Model file for the job. Use its own axes, mm. Face numbers are marked on the shaded views. A direction names the side the tool comes from. Give positions to 0.01 mm unless a question says otherwise; leave off trailing zeros. Loops run counter-clockwise (first coordinate to the right, second up) from the corner with the lowest first, then second, coordinate; pieces in that order, holes last. Notation, with made-up numbers: (-25.5, -37) -> (-3.5, -37) arc R16 ccw to (-3.5, -18) -> close; hole circle Ø10 at (-1.75, 74). An arc over 180 degrees is marked (long way). Use CSV: the item, a comma, the result in double quotes. Start each with the question number.
(1) Cut at A-A on x = 17. Write the cut outline in (y, z).
(2) Cut at D-D on z = 11. Write the cut outline in (x, y), then the cut area to 3 significant figures.
(3) Pull direction X, two halves, no side cores. Call the marked faces 3, 4 and 5: pulls with the +X half, pulls with the -X half, needs draft (parallel to the pull), parting line crosses it, or undercut.
(4) Flat gauge pins, fed straight in: pin 1 (2.5 mm diameter, centred on x = -15, z = -10, fed in from +Y); pin 2 (5.5 mm diameter, centred on x = -14.5, z = 11, fed in from -Y); pin 3 (5 mm diameter, centred on y = 14.5, z = -11.5, fed in from -X); pin 4 (8.5 mm diameter, centred on x = 7, z = -1, fed in from +Y). Where does each tip first touch, or does it go through?
(5) Cut at C-C on x = -14.5. Write the cut outline in (y, z), then the cut area to 3 significant figures.
(6) Drill centre lines: probe 1 along Z at (x, y) = (-8, 11); probe 2 along X at (y, z) = (1.5, 2.5); probe 3 along X at (y, z) = (1, -11). Where is each one in solid material? Low to high.
(7) 3-axis set-ups, long thin cutter, end or side, ignore diameter. For the marked faces 1 and 2: which of +Z, -Z, +X, -X, +Y, -Y reach the whole face in a straight line?
(8) Cut at B-B on y = 10.5. Write the cut outline in (x, z), then the cut area to 3 significant figures.
from build123d import *

# Parameters (mm, degrees)
SKETCH1_W           = 42
SKETCH1_H           = 28
BOSS_EXTRUDE1_DEPTH = 17
BOSS_EXTRUDE3_DEPTH = 0.8
SKETCH4_R           = 1.65
CUT_EXTRUDE1_DEPTH  = 10.8
SKETCH5_W           = 10
SKETCH5_H           = 5
CUT_EXTRUDE2_DEPTH  = 10.8
FILLET1_R           = 1.5
BOSS_EXTRUDE4_START = 1.5
SKETCH6_R           = 2.65
SKETCH6_R_2         = 1.65
BOSS_EXTRUDE4_DEPTH = 1.5


with BuildPart() as part:
    # Sketch1 → Boss-Extrude1 (new body)
    with BuildSketch(Plane(origin=(0, 0, 0), x_dir=(1, 0, 0), z_dir=(0, 1, 0))):
        Polygon((-22, 15), (-23.5, 4.326945416), (-23.5, -4.326945416), (-22, -15), (22, -15), (23.5, -4.326945416), (23.5, 4.326945416), (22, 15), align=None)
        Rectangle(SKETCH1_W, SKETCH1_H, mode=Mode.SUBTRACT)
    extrude(amount=BOSS_EXTRUDE1_DEPTH)

    # Sketch3 → Boss-Extrude3 (add)
    with BuildSketch(Plane.XZ):
        Polygon((-22, 15), (22, 15), (23.5, 4.326945416), (23.5, -4.326945416), (22, -15), (-22, -15), (-23.5, -4.326945416), (-23.5, 4.326945416), align=None)
    extrude(amount=BOSS_EXTRUDE3_DEPTH)

    # Sketch4 → Cut-Extrude1 (cut)
    with BuildSketch(Plane(origin=(0, 0, 0), x_dir=(1, 0, 0), z_dir=(0, 1, 0))):
        with Locations(Location((-14.5, 11, 0), (0, 0, 270))):
            Circle(SKETCH4_R)
        with Locations(Location((7.8, 11.302833977, 0), (0, 0, 270))):
            Circle(SKETCH4_R)
        with Locations(Location((-14.5, -11, 0), (0, 0, 270))):
            Circle(SKETCH4_R)
        with Locations(Location((7.8, -11.16509614, 0), (0, 0, 270))):
            Circle(SKETCH4_R)
    extrude(amount=-CUT_EXTRUDE1_DEPTH, mode=Mode.SUBTRACT)

    # Sketch5 → Cut-Extrude2 (cut)
    with BuildSketch(Plane.XY.offset(-14)):
        with Locations((16, 4)):
            Rectangle(SKETCH5_W, SKETCH5_H)
    extrude(amount=-CUT_EXTRUDE2_DEPTH, mode=Mode.SUBTRACT)

    # Fillet1
    fillet1_edges = [part.edges().sort_by_distance(p)[0] for p in [
        (11, 1.5, -14.5),
        (11, 6.5, -14.5),
    ]]
    fillet(fillet1_edges, radius=FILLET1_R)

    # Sketch6 → Boss-Extrude4 (add)
    # profile 1 of 4: a face of its own
    with BuildSketch(Plane(origin=(0, 0, 0), x_dir=(1, 0, 0), z_dir=(0, 1, 0)).offset(BOSS_EXTRUDE4_START)):
        with Locations(Location((-14.5, 11, 0), (0, 0, 270))):
            Circle(SKETCH6_R)
        with Locations(Location((-14.5, 11, 0), (0, 0, 270))):
            Circle(SKETCH6_R_2, mode=Mode.SUBTRACT)
    # profile 2 of 4: a face of its own
    with BuildSketch(Plane(origin=(0, 0, 0), x_dir=(1, 0, 0), z_dir=(0, 1, 0)).offset(BOSS_EXTRUDE4_START)):
        with Locations(Location((7.8, 11.302833977, 0), (0, 0, 270))):
            Circle(SKETCH6_R)
        with Locations(Location((7.8, 11.302833977, 0), (0, 0, 270))):
            Circle(SKETCH6_R_2, mode=Mode.SUBTRACT)
    # profile 3 of 4: a face of its own
    with BuildSketch(Plane(origin=(0, 0, 0), x_dir=(1, 0, 0), z_dir=(0, 1, 0)).offset(BOSS_EXTRUDE4_START)):
        with Locations(Location((7.8, -11.16509614, 0), (0, 0, 270))):
            Circle(SKETCH6_R)
        with Locations(Location((7.8, -11.16509614, 0), (0, 0, 270))):
            Circle(SKETCH6_R_2, mode=Mode.SUBTRACT)
    # profile 4 of 4: a face of its own
    with BuildSketch(Plane(origin=(0, 0, 0), x_dir=(1, 0, 0), z_dir=(0, 1, 0)).offset(BOSS_EXTRUDE4_START)):
        with Locations(Location((-14.5, -11, 0), (0, 0, 270))):
            Circle(SKETCH6_R)
        with Locations(Location((-14.5, -11, 0), (0, 0, 270))):
            Circle(SKETCH6_R_2, mode=Mode.SUBTRACT)
    extrude(amount=-BOSS_EXTRUDE4_DEPTH)


solid = part.part
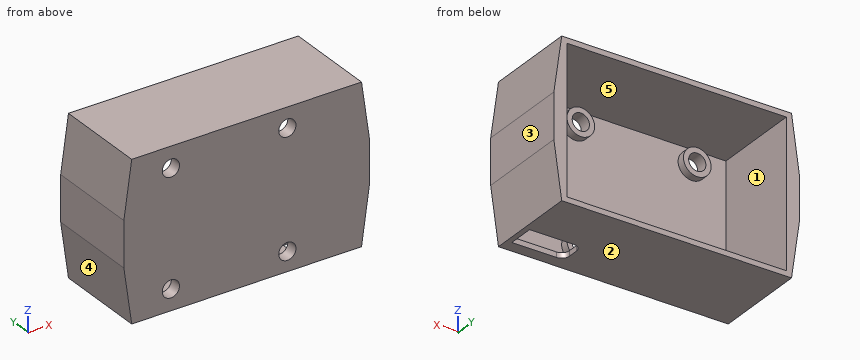
Check result:
1,outline,"(-0.8, -15) -> (1.5, -15) -> (1.5, -14) -> (0, -14) -> (0, 14) -> (17, 14) -> (17, 15) -> (-0.8, 15) -> close; (6.5, -15) -> (17, -15) -> (17, -14) -> (6.5, -14) -> close"
2,outline,"(-22.56, -0.8) -> (-16.15, -0.8) -> (-16.15, 1.5) -> (-17.15, 1.5) -> (-17.15, 0) -> (-21, 0) -> (-21, 17) -> (-22.56, 17) -> close; (-12.85, -0.8) -> (6.16, -0.8) -> (6.16, 1.5) -> (5.16, 1.5) -> (5.16, 0) -> (-11.85, 0) -> (-11.85, 1.5) -> (-12.85, 1.5) -> close; (9.44, -0.8) -> (22.56, -0.8) -> (22.56, 17) -> (21, 17) -> (21, 0) -> (10.44, 0) -> (10.44, 1.5) -> (9.44, 1.5) -> close"
2,area,"90.0 mm²"
3,face 3,"pulls with the +X half"
3,face 4,"pulls with the -X half"
3,face 5,"undercut"
4,pin 1,"y = 1.5"
4,pin 2,"y = -0.8"
4,pin 3,"x = -22.84"
4,pin 4,"y = 0"
5,outline,"(-0.8, -15) -> (17, -15) -> (17, -14) -> (0, -14) -> (0, -13.65) -> (1.5, -13.65) -> (1.5, -12.65) -> (-0.8, -12.65) -> close; (-0.8, -9.35) -> (1.5, -9.35) -> (1.5, -8.35) -> (0, -8.35) -> (0, 8.35) -> (1.5, 8.35) -> (1.5, 9.35) -> (-0.8, 9.35) -> close; (-0.8, 12.65) -> (1.5, 12.65) -> (1.5, 13.65) -> (0, 13.65) -> (0, 14) -> (17, 14) -> (17, 15) -> (-0.8, 15) -> close"
5,area,"58.7 mm²"
6,probe 1,"-15 to -14, 14 to 15"
6,probe 2,"-23.5 to -21, 21 to 23.5"
6,probe 3,"-22.56 to -21, -17.15 to -16.15, -12.85 to -11.85, 5.17 to 6.18, 9.42 to 10.43, 21 to 22.56"
7,face 1,"+Y"
7,face 2,"-Z, +X, -X, +Y, -Y"
8,outline,"(-23.5, -4.33) -> (-22, -15) -> (22, -15) -> (23.5, -4.33) -> (23.5, 4.33) -> (22, 15) -> (-22, 15) -> (-23.5, 4.33) -> close; hole (-21, -14) -> (21, -14) -> (21, 14) -> (-21, 14) -> close"
8,area,"202 mm²"
